Design review of the part shown in the three views and the two pictorial views. Dimensions are in mm from the part's minimum x, y and z. Give positions to 0.01 mm unless a question says otherwise; leave off trailing zeros. Loops run counter-clockwise (first coordinate to the right, second up) from the corner with the lowest first, then second, coordinate; pieces in that order, holes last. Notation, with made-up numbers: (87, -18.75) -> (106, -18.75) arc R18 ccw to (106, -11.75) -> close; hole circle Ø5 at (52, -4). An arc over 180 degrees is marked (long way). Answer as CSV lines item,"result".
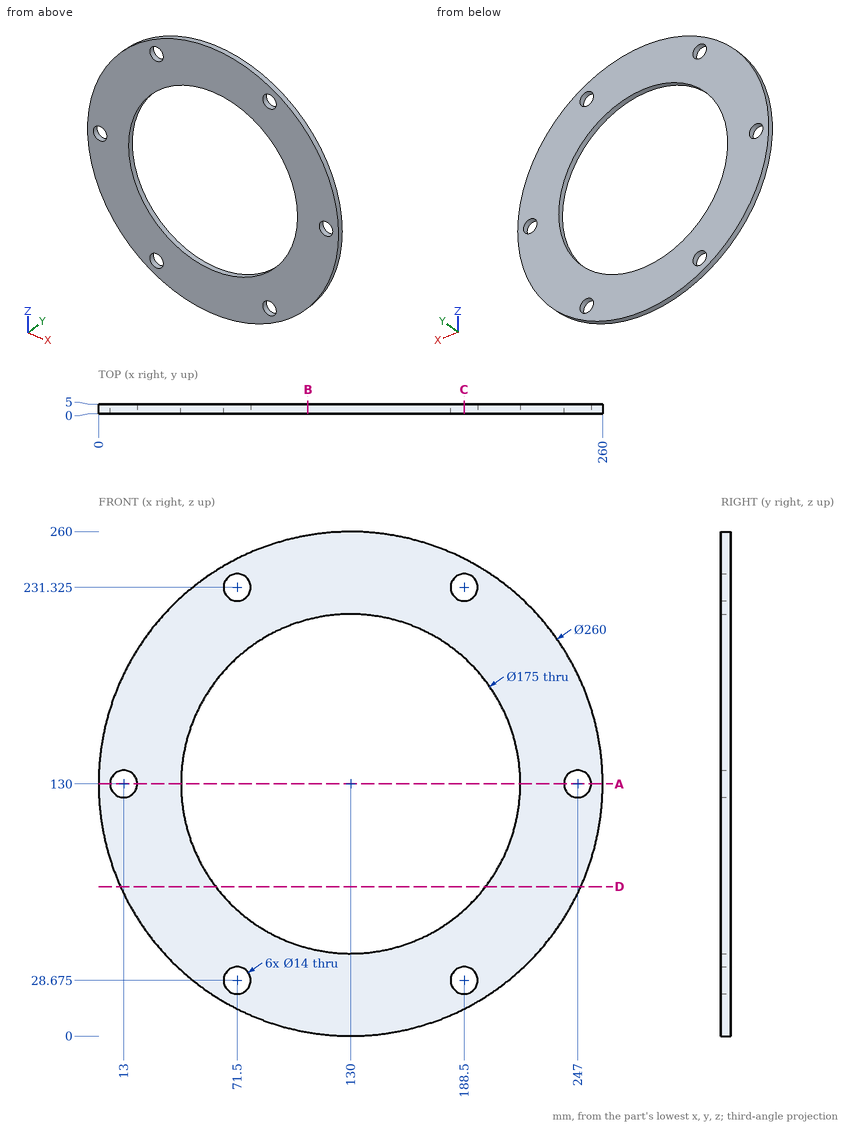
Q1. Clearance check with flat-ended pins moving along their axes: pin 1 Ø5 at (x, z) = (108.5, 212) entering from +Y; pin 2 Ø1 at (y, z) = (1.5, 188) entering from -X; pin 3 Ø2 at (x, y) = (93.5, 2.5) entering from +Z; pin 4 Ø1.5 at (y, z) = (2.5, 89) entering from +X. State where each tip first meets the part, or that it passes through.
Filled sheet:
pin 1,"passes through"
pin 2,"stops at x = 13.41"
pin 3,"stops at z = 255.06"
pin 4,"stops at x = 253.61"
Q2. To check wall thickness, follow probe 1 along Z at (x, y) = (130, 3.7); probe 2 along X at (y, z) = (4.2, 22.5); probe 3 along Z at (x, y) = (188.5, 3.1) (3 decimals). State the ranges of each line that lie inside material, in increasing order. Write a range as from..to.
Filled sheet:
probe 1,"z = 0..42.5, 217.5..260"
probe 2,"x = 56.9..68.2, 74.8..185.2, 191.8..203.1"
probe 3,"z = 13.906..21.675, 35.675..64.931, 195.069..224.325, 238.325..246.094"
Q3. We need section C-C, the plane x = 188.5. State the section outline as (y, z) points (3 decimals), and give its area (3 significant figures).
Filled sheet:
outline,"(0, 13.906) -> (5, 13.906) -> (5, 21.675) -> (0, 21.675) -> close; (0, 35.675) -> (5, 35.675) -> (5, 64.931) -> (0, 64.931) -> close; (0, 195.069) -> (5, 195.069) -> (5, 224.325) -> (0, 224.325) -> close; (0, 238.325) -> (5, 238.325) -> (5, 246.094) -> (0, 246.094) -> close"
area,"370 mm^2"
Q4. We need section A-A, the plane z = 130. State the section outline as (x, y) points, and give its area (3 significant figures).
Filled sheet:
outline,"(0, 0) -> (6, 0) -> (6, 5) -> (0, 5) -> close; (20, 0) -> (42.5, 0) -> (42.5, 5) -> (20, 5) -> close; (217.5, 0) -> (240, 0) -> (240, 5) -> (217.5, 5) -> close; (254, 0) -> (260, 0) -> (260, 5) -> (254, 5) -> close"
area,"285 mm^2"
Q5. We need section B-B, the plane x = 108. State the section outline as (y, z) points (3 decimals), and give its area (3 significant figures).
Filled sheet:
outline,"(0, 1.875) -> (5, 1.875) -> (5, 45.311) -> (0, 45.311) -> close; (0, 214.689) -> (5, 214.689) -> (5, 258.125) -> (0, 258.125) -> close"
area,"434 mm^2"
Q6. We need section D-D, the plane z = 77. State the section outline as (x, y) points, and give its area (3 significant figures).
Filled sheet:
outline,"(11.29, 0) -> (60.38, 0) -> (60.38, 5) -> (11.29, 5) -> close; (199.62, 0) -> (248.71, 0) -> (248.71, 5) -> (199.62, 5) -> close"
area,"491 mm^2"
